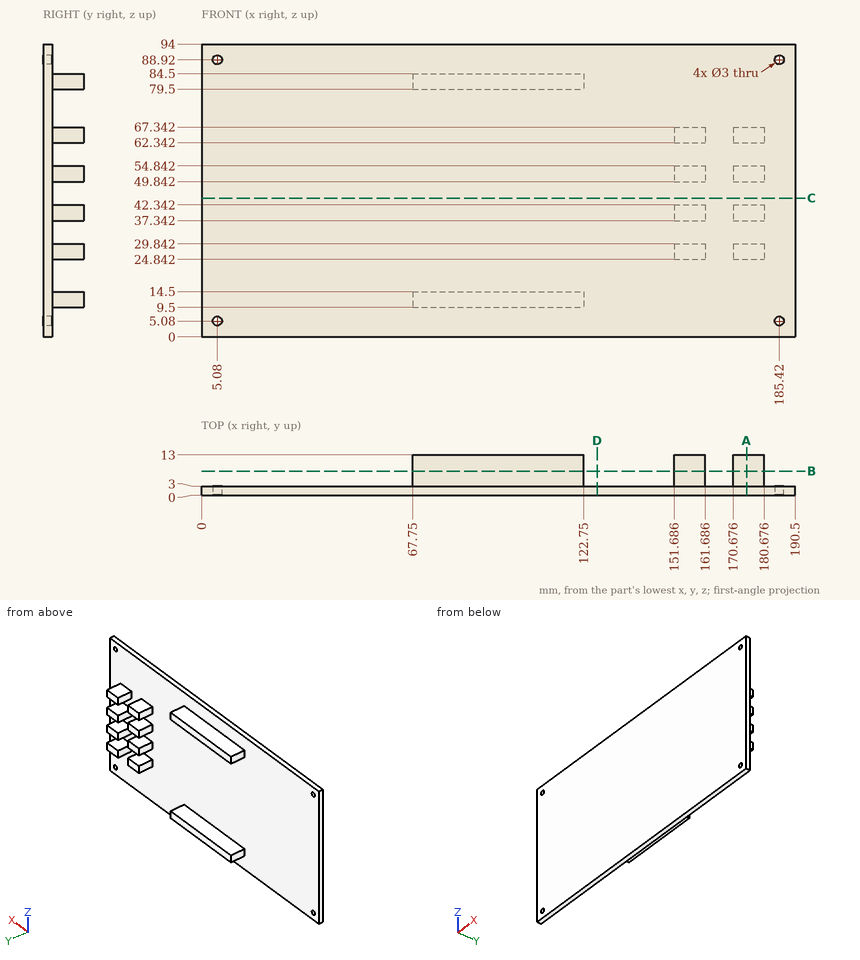
Geometry check sheet. Reference: drawing and pictorial views, mm from the part's lowest x, y, z. Give positions to 0.01 mm unless a question says otherwise; leave off trailing zeros. Order: outer loops, then holes, each group sorted by start corner. A loop starts at its lowest first (then second) coordinate and runs counter-clockwise, first axis right, second up. Notation, with made-up numbers: M -7,44 L 45,44 A19 ccw 45,80 Z; hole C -37,78.5 d5. An arc over 180 degrees is marked long. Answer in a Markdown table with one row per item. Add a question column.
Q1. Gauge pin test, flat ends, axial feed: pin 1 Ø2 at (x, z) = (33.5, 14) entering from -Y; pin 2 Ø6 at (x, z) = (51.5, 56.5) entering from +Y; pin 3 Ø2.5 at (y, z) = (9.5, 51.5) entering from +X; pin 4 Ø3 at (x, y) = (151, 7) entering from -Z. Record the tip position at first contact, or that the pin passes through.
Q2. Sectioned sample at C-C, the plane z = 44.5. Record the boundary of the cut face in (x, y).
Q3. Sectioned sample at A-A, the plane x = 175. Record the boundary of the cut face in (y, z).
Q4. Thickness scan on L1, parallel to Z at x = 185.42, y = 2.45; L2, parallel to X at y = 1.55, z = 88.92; L3, parallel to X at y = 5.25, z = 26 (1 decimal). Record the ranges inside material, lowest first.
Q5. Sectioned sample at D-D, the plane x = 127. Record the boundary of the cut face in (y, z).
Q6. Sectioned sample at B-B, the plane y = 7.75. Count the separate pieces of the cut face and the enclosed holes in it, and give its area (3 significant figures).
Verdict:
| question | item | result |
|---|---|---|
| 1 | pin 1 | y = 0 |
| 1 | pin 2 | y = 3 |
| 1 | pin 3 | x = 180.68 |
| 1 | pin 4 | z = 24.84 |
| 2 | outline | M 0,0 L 190.5,0 L 190.5,3 L 0,3 Z |
| 3 | outline | M 0,0 L 3,0 L 3,24.84 L 13,24.84 L 13,29.84 L 3,29.84 L 3,37.34 L 13,37.34 L 13,42.34 L 3,42.34 L 3,49.84 L 13,49.84 L 13,54.84 L 3,54.84 L 3,62.34 L 13,62.34 L 13,67.34 L 3,67.34 L 3,94 L 0,94 Z |
| 4 | L1 | 0 to 3.58, 6.58 to 87.42, 90.42 to 94 |
| 4 | L2 | 0 to 3.58, 6.58 to 183.92, 186.92 to 190.5 |
| 4 | L3 | 151.7 to 161.7, 170.7 to 180.7 |
| 5 | outline | M 0,0 L 3,0 L 3,94 L 0,94 Z |
| 6 | separate pieces | 10 |
| 6 | enclosed holes | 0 |
| 6 | area | 950 mm² |
